Part model, mm, in its own coordinate system. Face numbers are marked on the shaded views. A direction names the side the tool comes from. Round coordinates to 2 decimals unless told otherwise and drop trailing zeros. Order: outer loops, then holes, each group sorted by start corner. A loop starts at its lowest first (then second) coordinate and runs counter-clockwise, first axis right, second up. Notation, with made-up numbers: (48, -33) - (53, -33) arc R9 ccw to (53, -16) - close; hole circle Ø6 at (68.25, 48.5). An arc over 180 degrees is marked (long way). Answer as a JSON object with one key per item and string values.
Autodesk Inventor part; units mm, degrees
ref_plane "YZ Plane" through (0, 0, 0) normal (1, 0, 0) x (0, 1, 0)
ref_plane "XZ Plane" through (0, 0, 0) normal (0, 1, 0) x (-1, 0, 0)
ref_plane "XY Plane" through (0, 0, 0) normal (0, 0, 1) x (1, 0, 0)
sketch "草图1" plane through (0, 0, 0) normal (0, 0, 1) x (1, 0, 0)
  circle A0 centre (0, 0) radius 2.7
  circle A1 centre (0, 0) radius 1.6
  line L0 (0, 0) -> (0, 11.5707) construction
  line L1 (1.6293, 0) -> (1.6293, 11.5707)
  line L2 (-1.6293, 11.5707) -> (-1.6293, 0)
  arc A2 (-1.6293, 0) -> (1.6293, 0) centre (0, 0) ccw
  arc A3 (1.6293, 11.5707) -> (-1.6293, 11.5707) centre (0, 11.5707) ccw
  point P0 (0, 5.7853)
  point P1 (0, 13.2)
  point P2 (0, -2.7)
  point P3 (-1.6293, 2.153)
  point P4 (1.6293, 2.153)
  dimension "d0" = 5.4
  dimension "d1" = 3.2
  dimension "d2" = 15.9
extrude "拉伸1" add sketch "草图1" along normal blind 1.15 contours A0 L2 A2 L1 | L1 A2 L2 A0 | A0 L2 A3 L1 | A1
sketch "草图2" plane through (0, 0, 1.15) normal (0, 0, 1) x (1, 0, 0)
  circle A0 centre (0, 0) radius 1.95
  circle A1 centre (0, 0) radius 2.7
  dimension "d5" = 3.9
extrude "拉伸2" add sketch "草图2" along normal blind 2.3
sketch "草图3" plane through (0, 0, 1.15) normal (0, 0, 1) x (1, 0, 0)
  circle A0 centre (0, 11.5462) radius 0.5
  circle A1 centre (0, 9.1462) radius 0.5
  circle A2 centre (0, 6.85) radius 0.5
  circle A3 centre (0, 0) radius 1.95
  dimension "d8" = 1
  dimension "d9" = 1
  dimension "d10" = 1
  dimension "d12" = 6.85
  dimension "d13" = 2.4
extrude "拉伸3" cut sketch "草图3" against normal blind 2.3 contours A0 | A1 | A2
properties part number "摆臂"
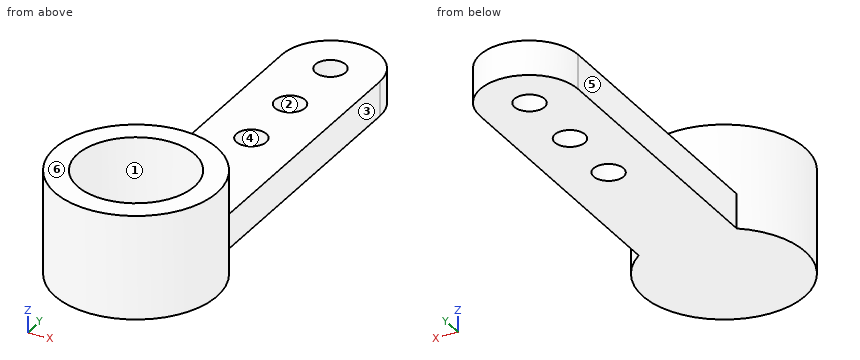
Item 1: Two-plate mould, pull along X, no slides. Class the marked faces 4, 5 and 6: pulls with the +X half, pulls with the -X half, needs draft (parallel to the pull), parting line crosses it, or undercut.
Taken from the geometry:
{"face 4": "undercut", "face 5": "pulls with the -X half", "face 6": "needs draft"}
Item 2: Cut at D-D (x = 0.65). Write the cut outline in (y, z), plus the area to 3 significant figures.
Taken from the geometry:
{"outline": "(-2.62, 0) - (13.06, 0) - (13.06, 1.15) - (2.62, 1.15) - (2.62, 3.45) - (1.84, 3.45) - (1.84, 1.15) - (-1.84, 1.15) - (-1.84, 3.45) - (-2.62, 3.45) - close", "area": "21.6 mm2"}
Item 3: Cut at B-B (x = 0). Write the cut outline in (y, z), plus the area to 3 significant figures.
Taken from the geometry:
{"outline": "(-2.7, 0) - (6.35, 0) - (6.35, 1.15) - (2.7, 1.15) - (2.7, 3.45) - (1.95, 3.45) - (1.95, 1.15) - (-1.95, 1.15) - (-1.95, 3.45) - (-2.7, 3.45) - close; (7.35, 0) - (8.65, 0) - (8.65, 1.15) - (7.35, 1.15) - close; (9.65, 0) - (11.05, 0) - (11.05, 1.15) - (9.65, 1.15) - close; (12.05, 0) - (13.2, 0) - (13.2, 1.15) - (12.05, 1.15) - close", "area": "18.3 mm2"}
Item 4: Cut at C-C (z = 0.4). Write the cut outline in (x, y).
Taken from the geometry:
{"outline": "(-1.63, 2.15) arc R2.7 ccw (long way) to (1.63, 2.15) - (1.63, 11.57) arc R1.63 ccw to (-1.63, 11.57) - close; hole circle Ø1 at (0, 6.85); hole circle Ø1 at (0, 9.15); hole circle Ø1 at (0, 11.55)"}
Item 5: Drop flat-ended pins along their axis: P1, Ø1.3, axis at y = 5, z = 0.5, coming from the -X side; P2, Ø1, axis at x = 0.5, z = 2, coming from the -Y side; P3, Ø0.6, axis at y = 7.5, z = 0.5, coming from the +X side; P4, Ø1, axis at x = 0, y = 5, coming from the +Z side. Give the stop position or say it passes through.
Taken from the geometry:
{"P1": "x = -1.63", "P2": "y = -2.7", "P3": "x = 1.63", "P4": "z = 1.15"}
Item 6: Cut at A-A (y = 6.85). Write the cut outline in (x, z), plus the area to 3 significant figures.
Taken from the geometry:
{"outline": "(-1.63, 0) - (-0.5, 0) - (-0.5, 1.15) - (-1.63, 1.15) - close; (0.5, 0) - (1.63, 0) - (1.63, 1.15) - (0.5, 1.15) - close", "area": "2.60 mm2"}
Item 7: Tool access for the marked faces 1, 2 and 3: list every direction of +Z, -Z, +X, -X, +Y, -Y with a clear straight run to the whole face (end or side of a thin tool).
Taken from the geometry:
{"face 1": "+Z", "face 2": "+Z, -Z", "face 3": "+Z, -Z, +X, +Y"}
Item 8: Probe L1, parallel to Y at x = 0, z = 0.8; L2, parallel to Y at x = 0, z = 2.8; L3, parallel to Y at x = 1.75, z = 3.25. List the from-to ranges inside material, lowest first. Write a range as from..to.
Taken from the geometry:
{"L1": "-2.7..6.35, 7.35..8.65, 9.65..11.05, 12.05..13.2", "L2": "-2.7..-1.95, 1.95..2.7", "L3": "-2.06..-0.86, 0.86..2.06"}
